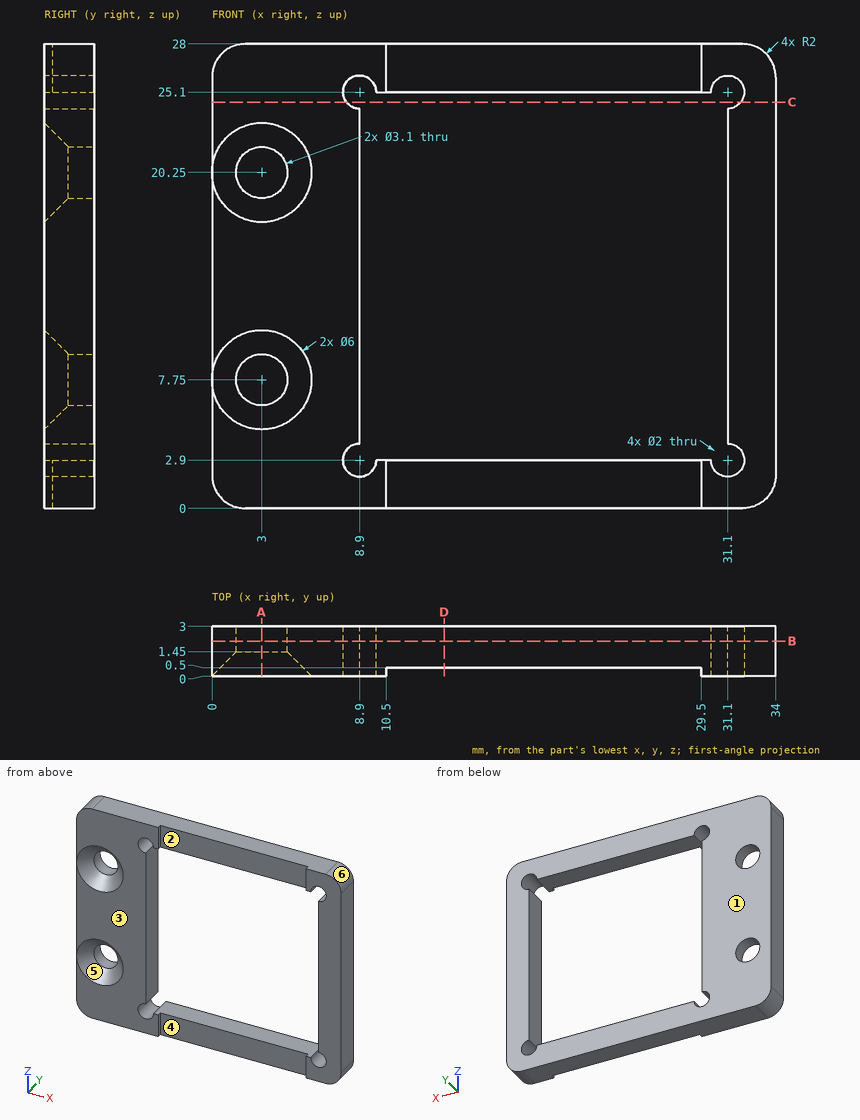
Print and shaded views of the part. All mm, measured from the part's lowest x, y and z. A direction names the side the tool comes from. Round coordinates to 2 decimals unless told otherwise and drop trailing zeros. Order: outer loops, then holes, each group sorted by start corner. A loop starts at its lowest first (then second) coordinate and runs counter-clockwise, first axis right, second up. Notation, with made-up numbers: (27, 80.25) - (78, 80.25) arc R26 cw to (78, 112.25) - close; hole circle Ø9 at (-19, 48). An arc over 180 degrees is marked (long way). Use a Markdown table: item, result.
1) Pull direction X, two halves, no side cores. Call the marked faces 3, 4, 5 and 6: pulls with the +X half, pulls with the -X half, needs draft (parallel to the pull), parting line crosses it, or undercut.
Recorded:
| item | result |
|---|---|
| face 3 | needs draft |
| face 4 | undercut |
| face 5 | undercut |
| face 6 | pulls with the +X half |
2) Saw through at D-D on x = 14. Write the cut outline in (y, z), and give its area (3 significant figures).
Recorded:
| item | result |
|---|---|
| outline | (0.5, 0) - (3, 0) - (3, 2.9) - (0.5, 2.9) - close; (0.5, 25.1) - (3, 25.1) - (3, 28) - (0.5, 28) - close |
| area | 14.5 mm² |
3) Tool access for the marked faces 1 and 2: list every direction of +Z, -Z, +X, -X, +Y, -Y with a clear straight run to the whole face (end or side of a thin tool).
Recorded:
| item | result |
|---|---|
| face 1 | +Z, -Z, +X, -X, +Y |
| face 2 | +Z, -Z, -Y |
4) Flat gauge pins, fed straight in: pin 1 Ø5 at (x, z) = (3, 20.25) entering from -Y; pin 2 Ø1 at (x, y) = (13.5, 2) entering from -Z. Where does each tip first touch, or does it go through?
Recorded:
| item | result |
|---|---|
| pin 1 | stops at y = 0.5 |
| pin 2 | stops at z = 0 |
5) Saw through at B-B on y = 2.1. Write the cut outline in (x, z), and give its area (3 significant figures).
Recorded:
| item | result |
|---|---|
| outline | (0, 2) arc R2 ccw to (2, 0) - (32, 0) arc R2 ccw to (34, 2) - (34, 26) arc R2 ccw to (32, 28) - (2, 28) arc R2 ccw to (0, 26) - close; hole circle Ø3.1 at (3, 7.75); hole circle Ø3.1 at (3, 20.25); hole (8.9, 3.9) arc R1 ccw (long way) to (9.9, 2.9) - (30.1, 2.9) arc R1 ccw (long way) to (31.1, 3.9) - (31.1, 24.1) arc R1 ccw (long way) to (30.1, 25.1) - (9.9, 25.1) arc R1 ccw (long way) to (8.9, 24.1) - close |
| area | 431 mm² |
6) Saw through at A-A on x = 3. Write the cut outline in (y, z), and give its area (3 significant figures).
Recorded:
| item | result |
|---|---|
| outline | (0, 0) - (3, 0) - (3, 6.2) - (1.45, 6.2) - (0, 4.75) - close; (0, 10.75) - (1.45, 9.3) - (3, 9.3) - (3, 18.7) - (1.45, 18.7) - (0, 17.25) - close; (0, 23.25) - (1.45, 21.8) - (3, 21.8) - (3, 28) - (0, 28) - close |
| area | 61.2 mm² |
7) Saw through at C-C on z = 24.5. Write the cut outline in (x, y), and give its area (3 significant figures).
Recorded:
| item | result |
|---|---|
| outline | (0, 0) - (8.1, 0) - (8.1, 3) - (0, 3) - close; (31.9, 0) - (34, 0) - (34, 3) - (31.9, 3) - close |
| area | 30.6 mm² |
8) Wall check: L1, parallel to Z at x = 3, y = 2.55; L2, parallel to X at y = 2.35, z = 22.75; L3, parallel to X at y = 1.9, z = 7. Give the ranges that are in metal, low to high.
Recorded:
| item | result |
|---|---|
| L1 | z = 0 to 6.2, 9.3 to 18.7, 21.8 to 28 |
| L2 | x = 0 to 8.9, 31.1 to 34 |
| L3 | x = 0 to 1.64, 4.36 to 8.9, 31.1 to 34 |
